from build123d import *

# Parameters (mm, degrees)
ANGULAR_ALUMINIO_ANGULAR_38MM_1_DEPTH = 280
CROQUIS8_W                            = 35.8
CROQUIS8_H                            = 250
CORTAR_EXTRUIR1_DEPTH                 = 4
CHAFL_N1_SIZE                         = 10
CROQUIS10_R                           = 2
CORTAR_EXTRUIR3_DEPTH                 = 10
CROQUIS12_R                           = 2
CORTAR_EXTRUIR4_DEPTH                 = 10


with BuildPart() as part:
    # Sketch11 → Angular ALUMINIO ANGULAR 38MM(1) (new body)
    with BuildSketch(Plane(origin=(0, 0, 0), x_dir=(-1, 0, 0), z_dir=(0, 1, 0))):
        with BuildLine():
            Line((0, 0), (0, 50.8))
            Line((0, 50.8), (0.00508, 50.8))
            ThreePointArc((0.00508, 50.8), (2.246551928, 49.871551928), (3.175, 47.63008))
            Line((3.175, 47.63008), (3.175, 7.9375))
            ThreePointArc((3.175, 7.9375), (4.569903955, 4.569903955), (7.9375, 3.175))
            Line((7.9375, 3.175), (47.63008, 3.175))
            ThreePointArc((47.63008, 3.175), (49.871551928, 2.246551928), (50.8, 0.00508))
            Line((50.8, 0.00508), (50.8, 0))
            Line((50.8, 0), (0, 0))
        make_face()
    extrude(amount=ANGULAR_ALUMINIO_ANGULAR_38MM_1_DEPTH)

    # Croquis8 → Cortar-Extruir1 (cut)
    with BuildSketch(Plane(origin=(0, 0, 0), x_dir=(0, 0, -1), z_dir=(1, 0, 0))):
        with Locations((-32.9, 140)):
            Rectangle(CROQUIS8_W, CROQUIS8_H)
    extrude(amount=-CORTAR_EXTRUIR1_DEPTH, mode=Mode.SUBTRACT)

    # Chaflán1
    chafl_n1_edges = [part.edges().sort_by_distance(p)[0] for p in [
        (-1.5875, 265, 15),
        (-1.5875, 15, 15),
    ]]
    chamfer(chafl_n1_edges, length=CHAFL_N1_SIZE)

    # Croquis10 → Cortar-Extruir3 (cut)
    with BuildSketch(Plane(origin=(0, 0, 0), x_dir=(-1, 0, 0), z_dir=(0, 0, -1))):
        with Locations((5.675, 41)):
            Circle(CROQUIS10_R)
        with Locations((5.675, 11)):
            Circle(CROQUIS10_R)
        with Locations((-44.325, 41)):
            Circle(CROQUIS10_R)
        with Locations((-44.325, 11)):
            Circle(CROQUIS10_R)
    extrude(amount=-CORTAR_EXTRUIR3_DEPTH, mode=Mode.SUBTRACT)

    # Croquis12 → Cortar-Extruir4 (cut)
    with BuildSketch(Plane(origin=(0, 0, 0), x_dir=(-1, 0, 0), z_dir=(0, 0, -1))):
        with Locations((5.675, 269)):
            Circle(CROQUIS12_R)
        with Locations((5.675, 239)):
            Circle(CROQUIS12_R)
    extrude(amount=-CORTAR_EXTRUIR4_DEPTH, mode=Mode.SUBTRACT)


solid = part.part
For this review, take the finished solid that the model builds, in its own axes (mm). A direction names the side the tool comes from. Give positions to 0.01 mm unless a question says otherwise; leave off trailing zeros. Loops run counter-clockwise (first coordinate to the right, second up) from the corner with the lowest first, then second, coordinate; pieces in that order, holes last. Notation, with made-up numbers: M 16,20 L 24,20 A25 cw 24,46 Z; hole C 62,66.5 d5. An arc over 180 degrees is marked long. Answer as a JSON object with one key per item and string values. Group by question number.
Q1. Tool access review of faces 4 (the flat face through (-14, 280, 3)), 5 (the flat face through (-2, 260, 20)), 6 (the flat face through (-3.175, 129, 13)): name each direction out of +Z, -Z, +X, -X, +Y, -Y from which nothing blocks a thin tool from reaching the whole face with its end or side.
Q2. Mouldability with a two-part tool opening along Y and no side actions: class faces 1 (the flat face through (-14, 0, 3)), 2 (the flat face through (0, 107, 14)), 3 (the flat face through (-2, 20, 20)) as +Y half, -Y half, draft (parallel to the pull), parting line (faces both ways), or undercut.
Q3. For probe 1 along Z at (x, y) = (-11.5, 210) (3 decimals); probe 2 along Z at (x, y) = (-2, 137.5); probe 3 along X at (y, z) = (64, 8) (3 decimals), list the stretches that pass through material, from the lowest coordinate up. Write a range as [from, to].
Q4. Add section C-C on x = -43. Give the boundary of the cut face in (y, z) (3 decimals).
Q5. Add section A-A on z = 30. Give the boundary of the cut face in (x, y) (3 decimals), and give its area (4 significant figures).
Q6. Insertion check: P1, Ø6, axis at x = -19, y = 134, coming from the +Z side (3 decimals); P2, Ø2.5, axis at x = -1.5, z = 41, coming from the -Y side; P3, Ø10, axis at y = 148.5, z = 11, coming from the -X side; P4, Ø2.5, axis at x = -2, y = 169.5, coming from the +Z side. Each pin has a flat end and moves straight along its axis. Give the tip position at first contact, or say it passes through.
Checked values:
{
 "1": {"face 4": "+Z, -Z, +X, -X, +Y", "face 5": "+Z, +X, -X", "face 6": "+Z, -X, +Y, -Y"},
 "2": {"face 1": "-Y half", "face 2": "draft", "face 3": "undercut"},
 "3": {"probe 1": "[0, 3.175]", "probe 2": "[0, 15]", "probe 3": "[-3.175, 0]"},
 "4": {"outline": "M 0,0 L 280,0 L 280,3.175 L 0,3.175 Z"},
 "5": {"outline": "M -3.175,0 L 0,0 L 0,15 L -3.175,15 Z; M -3.175,265 L 0,265 L 0,280 L -3.175,280 Z", "area": "95.25 mm²"},
 "6": {"P1": "z = 3.175", "P2": "y = 0", "P3": "x = -3.59", "P4": "z = 15"}
}
